The listing builds one solid part. Answer for the finished solid, in the listing's coordinates (mm). A direction names the side the tool comes from. Coordinates: 2 decimals unless noted, no trailing zeros. Order: outer loops, then holes, each group sorted by start corner. A loop starts at its lowest first (then second) coordinate and runs counter-clockwise, first axis right, second up. Notation, with made-up numbers: M -37,89 L -13,89 A20 ccw -13,111 Z; hole C -12,-10 d11. An arc over 180 degrees is marked long. One line per item, written item: value. Start each with the question number.
Q1. Determine the mould class of faces 3 (the conical face through (2.08, 0.65, -2.12)), 4 (the flat face through (0, 0, -12)), 5 (the flat face through (0, 0, -1.51)) for opening direction Y: pulls with the +Y half, pulls with the -Y half, needs draft (parallel to the pull), parting line crosses it, or undercut.
Q2. Each of these flat-tipped pins is pushed along its axis until it touches: pin 1 Ø3 at (x, z) = (2.5, -3) entering from -Y; pin 2 Ø1.5 at (x, z) = (-1.5, -9.5) entering from +Y; pin 3 Ø3 at (y, z) = (-3, -3) entering from -X. Where does it stop, or does it pass through?
Q3. Straight lines are drawn through the part: line 1 along Y through (x, z) = (0, -10.25); line 2 along Z through (x, y) = (1, -1.25); line 3 along Y through (x, z) = (1, -3.25). For each, find the intervals that lie inside material, in ascending order. Write a range as [from, to].
Q4. The part is cut by section A-A on z = -7.25. Give the vertices of the cut face in (x, y).
Q5. For faces 1 (the cylindrical face through (0, 2, -7)), 2 (the flat face through (0, 2, 0)), determine the directions among +Z, -Z, +X, -X, +Y, -Y from which every point of the face is accessible in a straight line to the end or side of a thin tool.
Autodesk Inventor part; units mm, degrees
ref_plane "MSC_PF1" through (0, 0, 0) normal (1, 0, 0) x (0, 1, 0)
ref_plane "MSC_PT1" through (0, 0, 0) normal (0, 0, -1) x (-1, 0, 0)
ref_plane "YZ Plane" through (0, 0, 0) normal (1, 0, 0) x (0, 1, 0)
sketch "Skizze1" plane through (0, 0, 0) normal (0, 1, 0) x (-1, 0, 0)
  point P0 (0, 0)
sketch "Skizze2" plane through (0, 0, 0) normal (0, 1, 0) x (-1, 0, 0)
  line L0 (-2, -12) -> (0, -12)
  line L1 (-2, -2.3) -> (-2, -12)
  line L2 (-4, -0.3) -> (-2, -2.3)
  line L3 (-4, 0) -> (-4, -0.3)
  line L4 (0, 0) -> (-4, 0)
  line L5 (0, -12) -> (0, 0)
  line L6 (0, -12) -> (0, 0)
  line L7 (0, -14.4) -> (0, 2.4)
  line L8 (0.8, 0) -> (-4.8, 0)
  dimension "d3" = 4
  dimension "d5" = 2
  dimension "d7" = 12
  dimension "ParC" = 0.3
  dimension "d22" = 0
  dimension "d23" = 0
  dimension "d43" = 45
revolve "Drehung1" add sketch "Skizze2" angle 360 about axis through (0, 0, -12) along (0, 0, -1)
fillet "Rundung1" radius 0.2 1 edges at (-2, 0, -2.3)
chamfer "Fase1" distance 0.35 angle 45 1 edges at (-2, 0, -12) measured on face at (-0.9288, -1.7713, -8.7943)
thread "Gewinde1"
ref_plane "MSC_PF1" through (0, 0, 0) normal (1, 0, 0) x (0, 1, 0)
ref_plane "MSC_PT1" through (0, 0, 0) normal (0, 0, -1) x (-1, 0, 0)
sketch "Skizze4" plane through (0, 0, 0) normal (0, 0, 1) x (1, 0, 0)
  circle A0 centre (0, 0) radius 2.25
  circle A1 centre (0, 0) radius 1.575
  line L0 (0, 0) -> (1.364, -0.7875)
  line L1 (0, 0) -> (1.364, 0.7875)
  line L2 (1.364, -0.7875) -> (2.25, 0)
  line L3 (2.25, 0) -> (1.364, 0.7875)
  line L4 (-5.6, 0) -> (5.6, 0)
  dimension "d45" = 4.5
  dimension "d44" = 3.15
  dimension "d46" = 30
  dimension "d47" = 30
extrude "Extrusion2" cut sketch "Skizze4" against normal blind 1.51 contours L4 A1 L3 | L2 A1 L4 | L0 L4 A1 | A1 L4 L1 picked at (0.948, -0.4421) picked at (0.948, 0.4421)
pattern_circular "Runde Anordnung1" count 6 over 360 about axis through (0, 0, 0) along (0, 0, -1) of "Extrusion2"
fillet "Rundung2" radius 0.5 12 edges at (-1.125, 1.9486, -0.755) (-1.364, 0.7875, -0.755) (0, 1.575, -0.755) (-2.25, 0, -0.755) (1.364, 0.7875, -0.755) (2.25, 0, -0.755) (1.125, 1.9486, -0.755) (1.364, -0.7875, -0.755) (1.125, -1.9486, -0.755) (-1.364, -0.7875, -0.755) (-1.125, -1.9486, -0.755) (0, -1.575, -0.755)
equation "\"d3\" = 0.5 * dk"
equation "\"d5\" = 0.5 * NND"
equation "\"d7\" = NLG"
equation "\"d43\" = 0.5 * ang"
equation "\"d18\" = r"
equation "\"d19\" = 0.5 * PTC"
equation "\"d39\" = 0.5 * PTC"
equation "\"NND\" = 4"
equation "\"PTC\" = 0.7"
equation "\"dk\" = 8"
equation "\"ParK\" = 2.3"
equation "\"ParS\" = 2.5"
equation "\"ParT\" = 1.8"
equation "\"r\" = 0.2"
equation "\"NLG\" = 12"
equation "\"ang\" = 90deg"
equation "\"THREADDIA\" = NND"
properties part number "DIN 7991 - M4x12" material "Stahl, weich"
Output:
1. face 3: parting line crosses it
1. face 4: needs draft
1. face 5: undercut
2. pin 1: stops at y = -1.93
2. pin 2: stops at y = 1.85
2. pin 3: stops at x = -1.36
3. line 1: y = [-2, 2]
3. line 2: z = [-12, -1.51]
3. line 3: y = [-1.73, 1.73]
4. outline: C 0,0 d4
5. face 1: -Z
5. face 2: +Z, +X, -X, +Y, -Y
